CAD build for the part. Positions are in the model's coordinates, mm. Coordinates: 2 decimals unless noted, no trailing zeros. Order: outer loops, then holes, each group sorted by start corner. A loop starts at its lowest first (then second) coordinate and runs counter-clockwise, first axis right, second up. Notation, with made-up numbers: (82, -10.5) - (86, -10.5) arc R19 cw to (86, 2.5) - close; hole circle Ø5 at (-19, 32). An arc over 180 degrees is marked (long way). Return JSON: item names as keys, results as strings.
from build123d import *

# Parameters (mm, degrees)
SKETCH1_W           = 46
SKETCH1_H           = 4
BOSS_EXTRUDE1_DEPTH = 13
CUT_EXTRUDE1_DEPTH  = 46
CUT_EXTRUDE2_DEPTH  = 46
CUT_EXTRUDE3_DEPTH  = 46


with BuildPart() as part:
    # Sketch1 → Boss-Extrude1 (new body)
    with BuildSketch(Plane.XY):
        with Locations((23, 2)):
            Rectangle(SKETCH1_W, SKETCH1_H)
    extrude(amount=BOSS_EXTRUDE1_DEPTH)

    # Sketch2 → Cut-Extrude1 (cut)
    with BuildSketch(Plane(origin=(46, 0, 0), x_dir=(0, 0, -1), z_dir=(1, 0, 0))):
        Polygon((-10.029675263, 4), (-13, 1.204486068), (-13, 4), align=None)
    extrude(amount=-CUT_EXTRUDE1_DEPTH, mode=Mode.SUBTRACT)

    # Sketch3 → Cut-Extrude2 (cut)
    with BuildSketch(Plane.XY.offset(13)):
        Polygon((46, 1.204486068), (43.471571356, 4), (46, 4), align=None)
    extrude(amount=-CUT_EXTRUDE2_DEPTH, mode=Mode.SUBTRACT)

    # Sketch4 → Cut-Extrude3 (cut)
    with BuildSketch(Plane.XY.offset(13)):
        Polygon((0, 1.204486068), (3.068298022, 4.272784089), (0, 4.272784089), align=None)
    extrude(amount=-CUT_EXTRUDE3_DEPTH, mode=Mode.SUBTRACT)


solid = part.part
Item 1: Wall check: L1, parallel to Z at x = 40.5, y = 3.4; L2, parallel to X at y = 2.4, z = 4.25; L3, parallel to Z at x = 30, y = 2.45. Give the ranges that are in metal, low to high. Write a range as [from, to].
Findings below:
{"L1": "z = [0, 10.67]", "L2": "x = [1.2, 44.92]", "L3": "z = [0, 11.68]"}
Item 2: Band-saw the part on C-C, the plane y = 1.6. List the corners of the cut face in (x, z).
Findings below:
{"outline": "(0.4, 0) - (45.64, 0) - (45.64, 12.58) - (0.4, 12.58) - close"}
Item 3: Band-saw the part on A-A, the plane x = 36. List the corners of the cut face in (y, z), then the cut area to 3 significant figures.
Findings below:
{"outline": "(0, 0) - (4, 0) - (4, 10.03) - (1.2, 13) - (0, 13) - close", "area": "47.8 mm²"}
Item 4: Drop a flat-ended pin along its axis: P1, Ø1.5, axis at y = 3.5, z = 9.5, coming from the +X side. Give the stop position or say it passes through.
Findings below:
{"P1": "stops at x = 44.6"}
Item 5: Band-saw the part on D-D, the plane y = 3.3. List the corners of the cut face in (x, z), then the cut area to 3 significant figures.
Findings below:
{"outline": "(2.1, 0) - (44.1, 0) - (44.1, 10.77) - (2.1, 10.77) - close", "area": "453 mm²"}
Item 6: Band-saw the part on B-B, the plane z = 3.25. List the corners of the cut face in (x, y), then the cut area to 3 significant figures.
Findings below:
{"outline": "(0, 0) - (46, 0) - (46, 1.2) - (43.47, 4) - (2.8, 4) - (0, 1.2) - close", "area": "177 mm²"}
